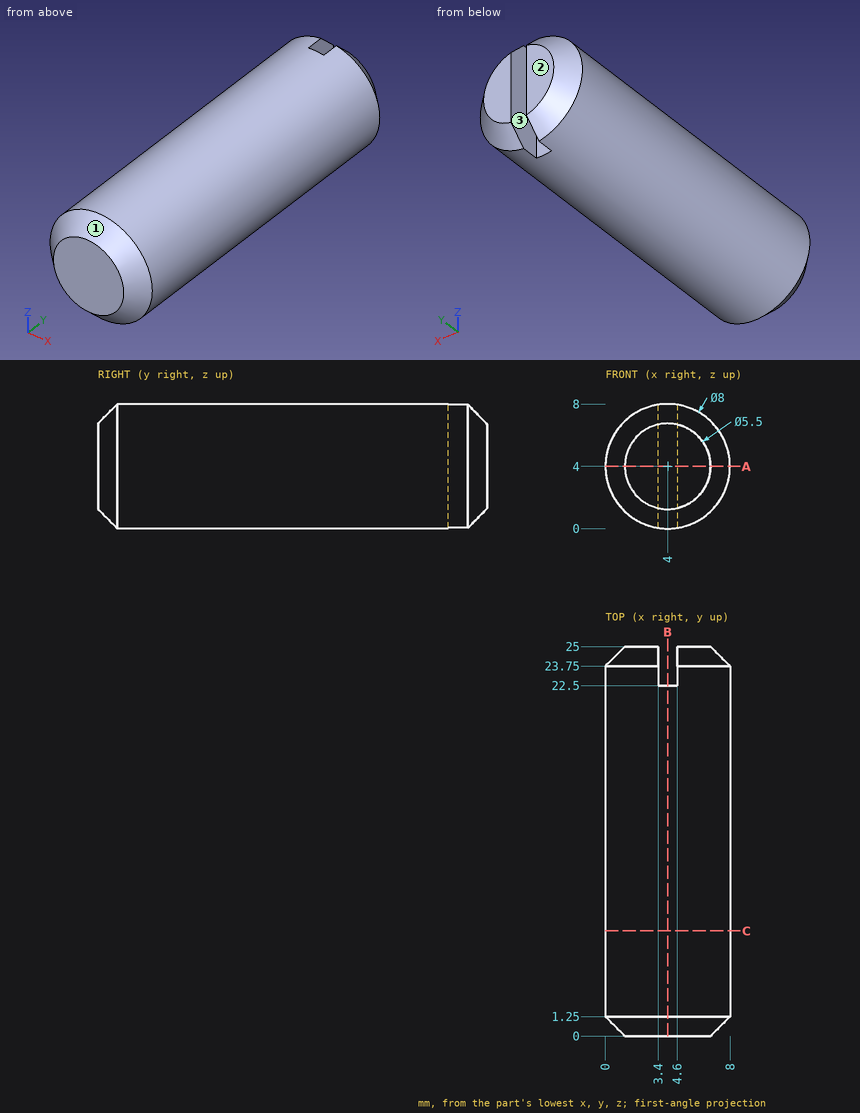
The figure shows three views and two pictorial views of one solid part (mm, origin at its lowest corner). Answer the questions. Round coordinates to 2 decimals unless told otherwise and drop trailing zeros. Write each loop counter-clockwise with the first axis right and the second up, starting at its lowest first coordinate (ties: lowest second). Pieces come first, ordered by that corner, then holes. Notation, with made-up numbers: M 43,61 L 86,61 A21 cw 86,79 Z; hole C 63,15 d9. An arc over 180 degrees is marked long. Write each question's results on one line, items separated by ' | '. Start each with the question number.
(1) Each of these flat-tipped pins is pushed along its axis until it touches: P1, Ø3, axis at y = 24.5, z = 5.5, coming from the -X side; P2, Ø0.6, axis at x = 4, z = 4, coming from the +Y side; P3, Ø2, axis at y = 24, z = 3.5, coming from the +X side; P4, Ø1, axis at y = 11, z = 7, coming from the -X side. Where does it stop, or does it pass through?
(2) The part is cut by section A-A, the plane z = 4. Write down the section's boundary in (x, y).
(3) Determine the mould class of the marked faces 1, 2 and 3 for opening direction X: +X half, -X half, draft (parallel to the pull), parting line (faces both ways), or undercut.
(4) The part is cut by section B-B, the plane x = 4. Write down the section's boundary in (y, z).
(5) Find the intervals of material crossed by line 1 (Y direction, x = 6.75, z = 6.75); line 2 (Y direction, x = 6.5, z = 1); line 3 (X direction, y = 19, z = 5), in increasing order.
(6) The part is cut by section C-C, the plane y = 6.75. Write down the section's boundary in (x, z).
Worked answers:
1) P1: stops at x = 0.01 | P2: stops at y = 22.5 | P3: stops at x = 8 | P4: stops at x = 0.88
2) outline: M 0,1.25 L 1.25,0 L 6.75,0 L 8,1.25 L 8,23.75 L 6.75,25 L 4.6,25 L 4.6,22.5 L 3.4,22.5 L 3.4,25 L 1.25,25 L 0,23.75 Z
3) face 1: parting line | face 2: draft | face 3: undercut
4) outline: M 0,1.25 L 1.25,0 L 22.5,0 L 22.5,8 L 1.25,8 L 0,6.75 Z
5) line 1: y = 1.14 to 23.86 | line 2: y = 1.16 to 23.84 | line 3: x = 0.13 to 7.87
6) outline: C 4,4 d8
